Geometry: see drawing. Coordinates: mm, zero at the bounding-box minimum. A direction names the side the tool comes from. Round coordinates to 2 decimals unless told otherwise and drop trailing zeros. Order: outer loops, then holes, each group sorted by start corner. A loop starts at its lowest first (then second) coordinate and runs counter-clockwise, first axis right, second up. Notation, with made-up numbers: (39, 25.5) -> (67, 25.5) arc R15 cw to (67, 51.5) -> close; hole circle Ø5 at (-1.5, -38.5). An arc over 180 degrees is marked (long way). Use a Markdown table: item, result.
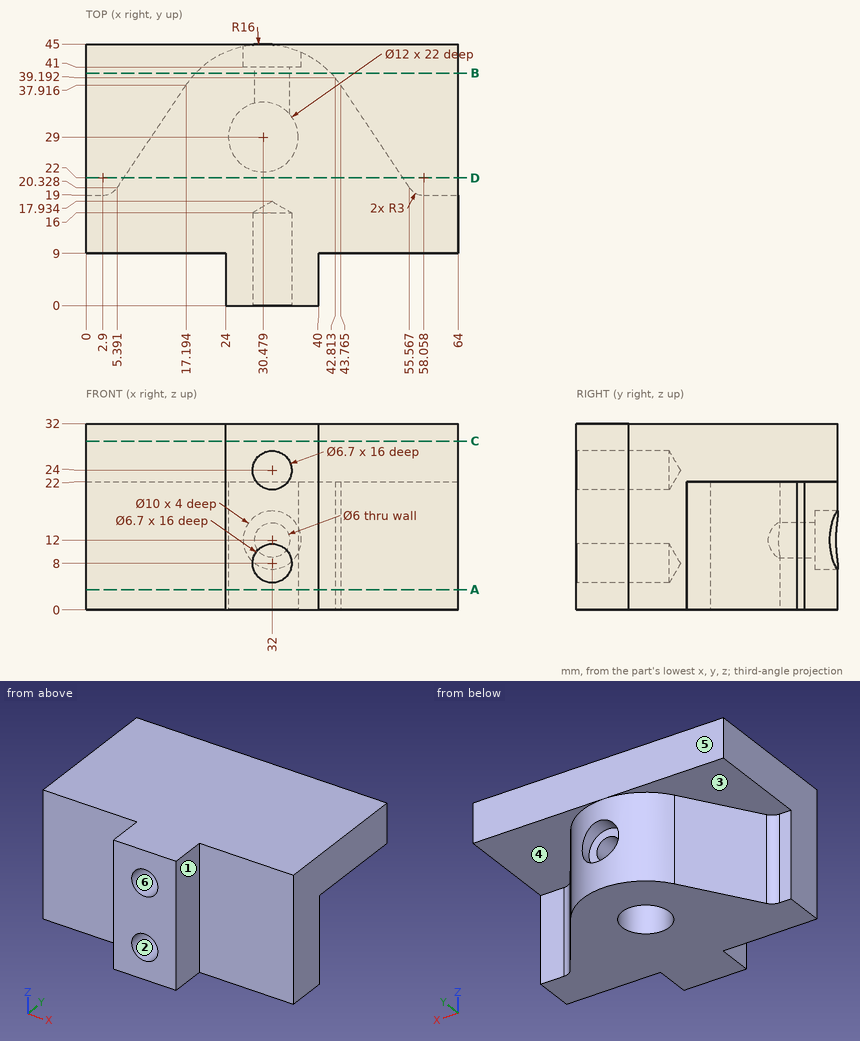
1) Cut plane D-D on y = 22. Return loops of the section in (x, z) (1 decimal), and give its area (3 significant figures).
Answer key:
| item | result |
|---|---|
| outline | (0, 22) -> (6.5, 22) -> (6.5, 0) -> (54.4, 0) -> (54.4, 22) -> (64, 22) -> (64, 32) -> (0, 32) -> close |
| area | 1,690 mm^2 |
2) Cut plane A-A on z = 3.5. Return loops of the section in (x, y) (1 decimal), and give its area (3 significant figures).
Answer key:
| item | result |
|---|---|
| outline | (0, 9) -> (24, 9) -> (24, 0) -> (40, 0) -> (40, 9) -> (64, 9) -> (64, 19) -> (58.1, 19) arc R3 cw to (55.6, 20.3) -> (43.8, 37.9) -> (42.8, 39.2) arc R16 ccw to (17.2, 37.9) -> (5.4, 20.3) arc R3 cw to (2.9, 19) -> (0, 19) -> close; hole circle Ø12 at (30.5, 29) |
| area | 1,550 mm^2 |
3) Contact query for flat-ended pins moving along their axis: P1, Ø1.8, axis at x = 61.5, z = 6.5, coming from the +Y side; P2, Ø10, axis at x = 51, z = 16, coming from the +Y side (1 decimal); P3, Ø8, axis at x = 32.5, z = 11.5, coming from the +Y side. Output: stop coordinate, or through.
Answer key:
| item | result |
|---|---|
| P1 | stops at y = 19 |
| P2 | stops at y = 34.6 |
| P3 | stops at y = 41 |
4) Cut plane C-C on z = 29. Return loops of the section in (x, y), and give its area (3 significant figures).
Answer key:
| item | result |
|---|---|
| outline | (0, 9) -> (24, 9) -> (24, 0) -> (40, 0) -> (40, 9) -> (64, 9) -> (64, 45) -> (0, 45) -> close |
| area | 2,450 mm^2 |
5) Ray query, probe 1 along Z at (x, y) = (32, 5); probe 2 along Z at (x, y) = (50.5, 39); probe 3 along X at (y, z) = (38.25, 12) (1 decimal). Return the intervals inside material, ascending.
Answer key:
| item | result |
|---|---|
| probe 1 | z = 0 to 4.65, 11.35 to 20.65, 27.35 to 32 |
| probe 2 | z = 22 to 32 |
| probe 3 | x = 17.4 to 29, 35 to 43.5 |
6) Set-up query: the marked faces 1, 2 and 3. Return all of +Z, -Z, +X, -X, +Y, -Y with unobstructed straight access to the full face (end or side cutting, diameter ignored); none if empty.
Answer key:
| item | result |
|---|---|
| face 1 | +Z, -Z, +X, -Y |
| face 2 | -Y |
| face 3 | -Z, -X, +Y |
7) Cut plane B-B on y = 40. Return loops of the section in (x, z), and give its area (3 significant figures).
Answer key:
| item | result |
|---|---|
| outline | (0, 22) -> (18.86, 22) -> (18.86, 0) -> (42.1, 0) -> (42.1, 22) -> (64, 22) -> (64, 32) -> (0, 32) -> close; hole circle Ø6 at (32, 12) |
| area | 1,120 mm^2 |
8) Draft query along Z for the marked faces 4, 5 and 6. Return one class per face: released by +Z, released by -Z, zero draft, split by the parting line, or undercut.
Answer key:
| item | result |
|---|---|
| face 4 | released by -Z |
| face 5 | zero draft |
| face 6 | undercut |
